Design review of the part built by this model. Coordinates are the model's own, in mm. Give positions to 0.01 mm unless a question says otherwise; leave off trailing zeros. Loops run counter-clockwise (first coordinate to the right, second up) from the corner with the lowest first, then second, coordinate; pieces in that order, holes last. Notation, with made-up numbers: (-30.5, -6) -> (-8.5, -6) arc R11 cw to (-8.5, 10) -> close; hole circle Ø9 at (57, 31). An arc over 180 degrees is marked (long way). Answer as CSV lines item,"result".
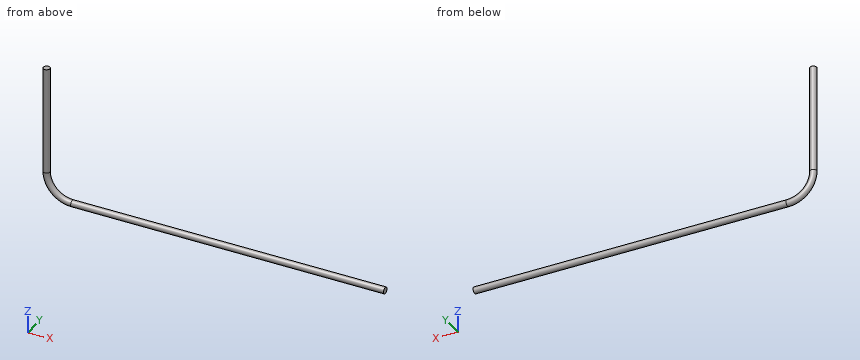
Autodesk Inventor part; units mm, degrees
ref_plane "Work Plane1" through (76.2, 0, 0) normal (1, 0, 0) x (0, 1, 0)
ref_plane "XZ Plane" through (0, 0, 0) normal (0, 1, 0) x (-1, 0, 0)
ref_plane "XY Plane" through (0, 0, 0) normal (0, 0, 1) x (1, 0, 0)
sketch "Sketch2" plane through (0, 0, 0) normal (0, 0, 1) x (1, 0, 0)
  circle A0 centre (0, 0) radius 9.525
  dimension "d3" = 19.05
extrude "Extrusion2" add sketch "Sketch2" against normal blind 317.5
ref_plane "Work Plane1" through (76.2, 0, 0) normal (1, 0, 0) x (0, 1, 0)
sketch "Sketch9" plane through (76.2, 0, 0) normal (1, 0, 0) x (0, 1, 0)
  line L0 (-9.525, -317.5) -> (9.525, -317.5)
  circle A0 centre (0, -393.7) radius 9.525
  line L1 (0, -317.5) -> (0, -393.7) construction
  point P0 (0, 0)
  dimension "d17" = 19.05
  dimension "d18" = 76.2
extrude "Extrusion4" add sketch "Sketch9" along normal blind 927.1
sketch "Sketch11" plane through (0, 0, -317.5) normal (0, 0, -1) x (-1, 0, 0)
  circle A0 centre (0, 0) radius 9.525
sketch "Sketch12" plane through (0, 0, 0) normal (0, 1, 0) x (-1, 0, 0)
  line L0 (-76.2, -403.225) -> (-76.2, -384.175)
  line L1 (-9.525, -317.5) -> (9.525, -317.5)
  arc A0 (-76.2, -393.7) -> (0, -317.5) centre (-76.2, -317.5) ccw
  point P0 (0, 0)
  dimension "d21" = 76.2
sweep "Sweep2" add profiles "Sketch11" path "Sketch12" path curves A0
equation "\"d3\" = tubeD"
equation "\"d17\" = tubeD"
equation "\"d18\" = tubeTurnR"
equation "\"d21\" = tubeTurnR"
equation "\"d4\" = tubeTurnR"
equation "\"wallThick\" = 44.45"
equation "\"roomWidth\" = 3048"
equation "\"roomDepth\" = 3657.6"
equation "\"roomHeight\" = 2438.4"
equation "\"doorWidth\" = 895.35"
equation "\"doorHeight\" = 2108.2"
equation "\"doorX\" = 774.7"
equation "\"doorY\" = 88.9"
equation "\"doorLip\" = 76.2"
equation "\"doorThick\" = 57.15"
equation "\"tubeTurnR\" = 76.2"
equation "\"tubeD\" = 19.05"
properties part number "left_tube_0"
Q1. To check wall thickness, follow probe 1 along X at (y, z) = (-1, -303); probe 2 along Z at (x, y) = (165.5, -1.5); probe 3 along X at (y, z) = (2, -196). State the ranges of each line that lie inside material, in increasing order. Write a range as from..to.
Filled sheet:
probe 1,"x = -9.47..9.47"
probe 2,"z = -403.11..-384.29"
probe 3,"x = -9.31..9.31"
Q2. We need section A-A, the plane y = 0. State the section outline as (x, z) points (3 decimals), and give its area (3 significant figures).
Filled sheet:
outline,"(-9.525, -317.5) arc R85.725 ccw to (76.2, -403.225) -> (1003.3, -403.225) -> (1003.3, -384.175) -> (76.2, -384.175) arc R66.675 cw to (9.525, -317.5) -> (9.525, 0) -> (-9.525, 0) -> close"
area,"26,000 mm^2"
Q3. Clearance check with flat-ended pins moving along their axes: pin 1 Ø8 at (x, y) = (465.5, -7) entering from -Z; pin 2 Ø8 at (y, z) = (-2, -237) entering from +X (3 decimals); pin 3 Ø5 at (y, z) = (7, -303) entering from +X (3 decimals). State where each tip first meets the part, or that it passes through.
Filled sheet:
pin 1,"stops at z = -402.74"
pin 2,"stops at x = 9.525"
pin 3,"stops at x = 8.395"
Q4. We need section B-B, the plane z = -71. State the section outline as (x, y) points (3 decimals).
Filled sheet:
outline,"circle Ø19.05 at (0, 0)"
Q5. We need section C-C, the plane x = 423. State the section outline as (y, z) points (3 decimals).
Filled sheet:
outline,"circle Ø19.05 at (0, -393.7)"
